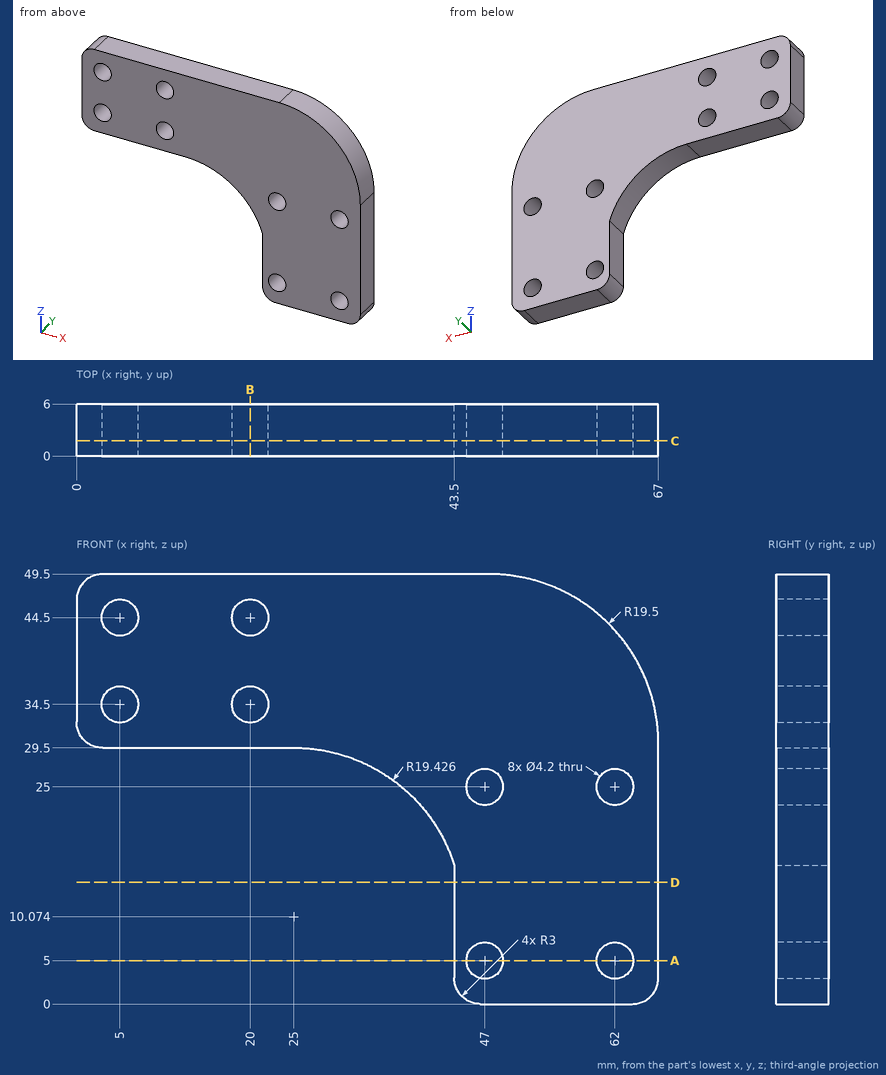
Could you check a few things on this drawing? It's one solid part, dimensions in mm from its lowest x, y, z. Coordinates: 2 decimals unless noted, no trailing zeros. Write each loop counter-clockwise with the first axis right and the second up, starting at its lowest first coordinate (ties: lowest second). Pieces come first, ordered by that corner, then holes.
Q1. Please list where these lines run through material, in increasing order: L1, parallel to Z at x = 5, y = 3.9; L2, parallel to X at y = 2.65, z = 5; L3, parallel to X at y = 3.1, z = 25.
Results found:
L1: z = 29.5 to 32.4, 36.6 to 42.4, 46.6 to 49.5
L2: x = 43.5 to 44.9, 49.1 to 59.9, 64.1 to 67
L3: x = 37.43 to 44.9, 49.1 to 59.9, 64.1 to 67
Q2. For P1, Ø3, axis at y = 4, z = 11.5, coming from the -X side, with a flat end and sliding along its axis, tell me the tip position at first contact or that it passes through.
Results found:
P1: stops at x = 43.5
Q3. Imagine slicing it at A-A, the plane z = 5. List the corners of the cut face in (x, y) for me, plus the area to 3 significant figures.
Results found:
outline: (43.5, 0) - (44.9, 0) - (44.9, 6) - (43.5, 6) - close; (49.1, 0) - (59.9, 0) - (59.9, 6) - (49.1, 6) - close; (64.1, 0) - (67, 0) - (67, 6) - (64.1, 6) - close
area: 90.6 mm2
Q4. Imagine slicing it at D-D, the plane z = 14. List the corners of the cut face in (x, y) for me, plus the area to 3 significant figures.
Results found:
outline: (43.5, 0) - (67, 0) - (67, 6) - (43.5, 6) - close
area: 141 mm2
Q5. Imagine slicing it at B-B, the plane x = 20. List the corners of the cut face in (y, z) for me, plus the area to 3 significant figures.
Results found:
outline: (0, 29.5) - (6, 29.5) - (6, 32.4) - (0, 32.4) - close; (0, 36.6) - (6, 36.6) - (6, 42.4) - (0, 42.4) - close; (0, 46.6) - (6, 46.6) - (6, 49.5) - (0, 49.5) - close
area: 69.6 mm2
Q6. Imagine slicing it at C-C, the plane y = 1.75. Count the separate pieces of the cut face and the enclosed holes in it, plus the area to 3 significant figures.
Results found:
separate pieces: 1
enclosed holes: 8
area: 1,900 mm2
